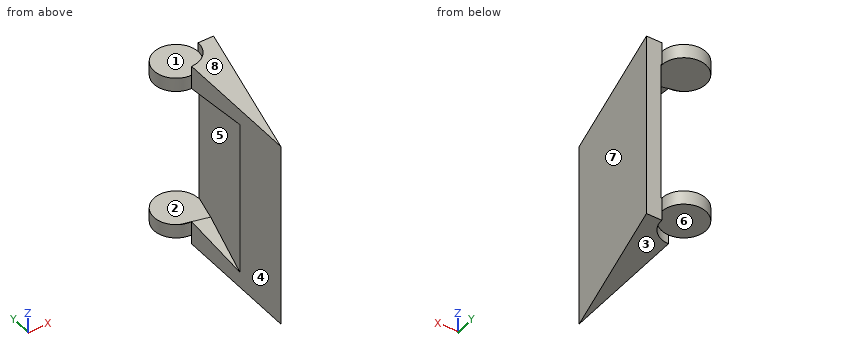
Autodesk Inventor part; units mm, degrees
ref_plane "YZ Plane" through (0, 0, 0) normal (1, 0, 0) x (0, 1, 0)
ref_plane "XZ Plane" through (0, 0, 0) normal (0, 1, 0) x (-1, 0, 0)
ref_plane "XY Plane" through (0, 0, 0) normal (0, 0, 1) x (1, 0, 0)
sketch "Sketch1" plane through (0, 0, 0) normal (0, 0, 1) x (1, 0, 0)
  line L0 (0, 50.8) -> (0, -50.8)
  line L1 (0, -50.8) -> (25.4, 50.8)
  line L2 (25.4, 50.8) -> (0, 50.8)
  point P0 (0, 0)
  point P1 (0, 0)
  dimension "d0" = 101.6
  dimension "d2" = 25.4
extrude "Extrusion1" add sketch "Sketch1" along normal mid plane 127
sketch "Sketch2" plane through (0, 0, 0) normal (0, 0, 1) x (1, 0, 0)
  line L0 (0, 50.8) -> (0, -50.8)
  circle A0 centre (0, 50.8) radius 15
  point P0 (0, 0)
  dimension "d5" = 30
extrude "Extrusion2" add sketch "Sketch2" along normal mid plane 114.3
sketch "Sketch3" plane through (0, 0, 63.5) normal (0, 0, 1) x (1, 0, 0)
  line L0 (0, 50.8) -> (0, -50.8)
  line L1 (0, 50.8) -> (25.4, 50.8)
  arc A0 (0, 35.8) -> (15, 50.8) centre (0, 50.8) ccw
  arc A1 (15, 50.8) -> (0, 35.8) centre (0, 50.8) ccw
  point P0 (0, 0)
extrude "Extrusion3" cut sketch "Sketch3" against normal up to surface (6.35 mm away) contours L1 A0 L0
mirror "Mirror1" about plane through (0, 0, 0) normal (0, 0, 1) of "Extrusion3"
ref_plane "Work Plane1" through (14.5521, 47.162, 0) normal (0.9701425, -0.2425356, 0) x (0.2425356, 0.9701425, 0)
sketch "Sketch4" plane through (14.5521, 47.162, 0) normal (0.9701425, -0.2425356, 0) x (0.2425356, 0.9701425, 0)
  line L0 (15, -57.15) -> (15, 57.15)
  line L1 (15, 47.625) -> (-14.5521, 47.625)
  line L2 (-14.5521, 47.625) -> (-98.5665, 57.15)
  line L3 (-98.5665, -63.5) -> (-98.5665, 63.5)
  line L4 (15, 0) -> (-98.5665, 0) construction
  line L5 (15, 57.15) -> (-15, 57.15) construction
  line L6 (-15, -57.15) -> (-15, 57.15) construction
  line L7 (-14.5521, 57.15) -> (-14.5521, -57.15) construction
  line L8 (15, -47.625) -> (-14.5521, -47.625)
  line L9 (-14.5521, -47.625) -> (-98.5665, -57.15)
  line L10 (15, 47.625) -> (15, -47.625)
  line L11 (-98.5665, 57.15) -> (-98.5665, -57.15)
  point P0 (-49.2832, 0)
  point P1 (3.638, 57.15)
  dimension "d10" = 6.35
  dimension "d11" = 9.525
extrude "Extrusion4" cut sketch "Sketch4" against normal through all
properties part number "NASA-20-ARM-SH-01"
Could you check a few things on this model? Use its own coordinates, in mm. Face numbers are marked on the shaded views. A direction names the side the tool comes from. Coordinates: 2 decimals unless noted, no trailing zeros. Order: outer loops, then holes, each group sorted by start corner. A loop starts at its lowest first (then second) coordinate and runs counter-clockwise, first axis right, second up. Notation, with made-up numbers: (-36, 33.25) -> (14, 33.25) arc R16 cw to (14, 54.25) -> close; hole circle Ø8 at (74, 73.5). An arc over 180 degrees is marked (long way). One line per item, written item: value. Start each with the question number.
1) Which directions (+Z, -Z, +X, -X, +Y, -Y) give clear straight access to the entire face, cutting with the end or side of a thin tool? Please do the marked faces 1, 2, 3 and 4.
2) Imagine slicing it at C-C on z = 25.5. List the corners of the cut face in (x, y) for me, plus the area to 3 significant figures.
3) I'm going to push flat-ended pins straight in: pin 1 (1 mm diameter, centred on y = 47, z = -35.5, fed in from -X); pin 2 (2 mm diameter, centred on y = 1, z = -31, fed in from +X); pin 3 (9 mm diameter, centred on x = -4, y = 43, fed in from -Z). Where does each tip first touch, or does it pass through?
4) Imagine slicing it at B-B on x = 3. List the corners of the cut face in (y, z) for me (3 decimals), plus the area to 3 significant figures.
5) If I drill on L1, parallel to Z at x = -1, y = 47.5 (3 decimals); L2, parallel to Z at x = 2, y = 11; L3, parallel to X at y = 30, z = 57.5, over which ranges is the centre line in solid material (lowest first)? Write a range as [from, to].
6) Imagine slicing it at D-D on y = 45.5. List the corners of the cut face in (x, z) for me (3 decimals).
7) We'd pull the mould along Z, two halves only. Please class the marked faces 5, 6, 7 and 8: +Z half, -Z half, draft (parallel to the pull), parting line (faces both ways), or undercut.
8) Imagine slicing it at A-A on y = 24.5. List the corners of the cut face in (x, z) for me (3 decimals), plus the area to 3 significant figures.
Answer list:
1. face 1: +Z, -X, +Y
1. face 2: -X, +Y
1. face 3: -Z, +X, -X, +Y, -Y
1. face 4: +Z, -Z, -X, -Y
2. outline: (0, -50.8) -> (25.4, 50.8) -> (15.46, 50.8) -> (0, -11.05) -> close
2. area: 812 mm2
3. pin 1: stops at x = 14.39
3. pin 2: stops at x = 13.2
3. pin 3: stops at z = -57.15
4. outline: (-38.8, -63.5) -> (36.103, -63.5) -> (36.103, -57.15) -> (65.497, -57.15) -> (65.497, -47.625) -> (35.05, -47.625) -> (0.954, -51.375) -> (0.954, 51.375) -> (35.05, 47.625) -> (65.497, 47.625) -> (65.497, 57.15) -> (36.103, 57.15) -> (36.103, 63.5) -> (-38.8, 63.5) -> close
4. area: 6,600 mm2
5. L1: z = [-57.15, -47.625], [47.625, 57.15]
5. L2: z = [-63.5, -50.3], [50.3, 63.5]
5. L3: x = [0, 20.2]
6. outline: (-14.032, -57.15) -> (14.032, -57.15) -> (14.032, -63.5) -> (24.075, -63.5) -> (24.075, 63.5) -> (14.032, 63.5) -> (14.032, 57.15) -> (-14.032, 57.15) -> (-14.032, 47.625) -> (14.137, 47.625) -> (14.137, -47.625) -> (-14.032, -47.625) -> close
7. face 5: undercut
7. face 6: -Z half
7. face 7: draft
7. face 8: +Z half
8. outline: (0, -63.5) -> (18.825, -63.5) -> (18.825, 63.5) -> (0, 63.5) -> (0, 48.868) -> (8.887, 48.624) -> (8.887, -48.624) -> (0, -48.868) -> close
8. area: 1,520 mm2
